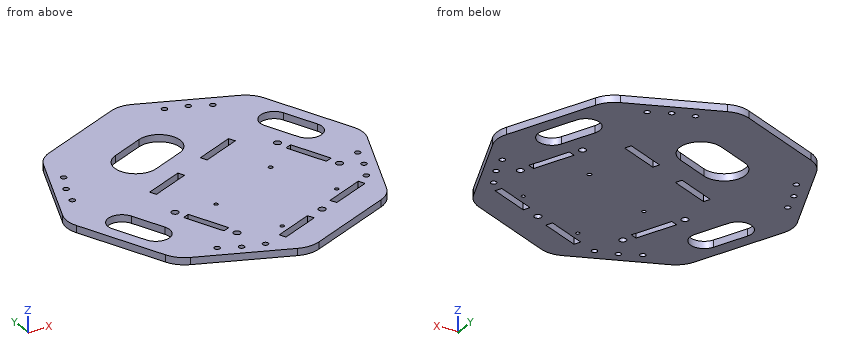
from build123d import *

# Parameters (mm, degrees)
SKETCH_1_R      = 2
SKETCH_1_R_2    = 2.5
SKETCH_1_R_3    = 1.35
SKETCH_1_R_4    = 1.5
EXTRUDE_1_DEPTH = 5
FILLET_1_R      = 20


with BuildPart() as part:
    # 草图1 → 凸台-拉伸1 (new body)
    with BuildSketch(Plane.XY):
        Polygon((0, 108.239220029), (-76.536686473, 76.536686473), (-108.239220029, 0), (-76.536686473, -76.536686473), (0, -108.239220029), (76.536686473, -76.536686473), (108.239220029, 0), (76.536686473, 76.536686473), align=None)
        with Locations((-35.206875778, -84.996916991)):
            Circle(SKETCH_1_R, mode=Mode.SUBTRACT)
        with Locations((84.996916991, -35.206875778)):
            Circle(SKETCH_1_R, mode=Mode.SUBTRACT)
        with Locations((35.206875778, 84.996916991)):
            Circle(SKETCH_1_R, mode=Mode.SUBTRACT)
        with Locations((-84.996916991, 35.206875778)):
            Circle(SKETCH_1_R, mode=Mode.SUBTRACT)
        with Locations((-45.41571145, -25.847352929)):
            Circle(SKETCH_1_R_2, mode=Mode.SUBTRACT)
        with Locations((-27.812273562, -68.345811425)):
            Circle(SKETCH_1_R_2, mode=Mode.SUBTRACT)
        with Locations((55.287157593, 15.865141198)):
            Circle(SKETCH_1_R_2, mode=Mode.SUBTRACT)
        with Locations((72.890595482, -26.633317297)):
            Circle(SKETCH_1_R_2, mode=Mode.SUBTRACT)
        with Locations((32.106246769, -70.586552674)):
            Circle(SKETCH_1_R_2, mode=Mode.SUBTRACT)
        with Locations((-18.756154363, -30.499289721)):
            Circle(SKETCH_1_R_3, mode=Mode.SUBTRACT)
        with Locations((-0.004666177, -75.769386814)):
            Circle(SKETCH_1_R_3, mode=Mode.SUBTRACT)
        with Locations((34.828858522, -8.303650644)):
            Circle(SKETCH_1_R_4, mode=Mode.SUBTRACT)
        with Locations((53.580346708, -53.573747737)):
            Circle(SKETCH_1_R_3, mode=Mode.SUBTRACT)
        with Locations((89.588318422, -20.926853617)):
            Circle(SKETCH_1_R, mode=Mode.SUBTRACT)
        with Locations((-20.926853617, -89.588318422)):
            Circle(SKETCH_1_R, mode=Mode.SUBTRACT)
        with Locations((-89.588318422, 20.926853617)):
            Circle(SKETCH_1_R, mode=Mode.SUBTRACT)
        with Locations((20.926853617, 89.588318422)):
            Circle(SKETCH_1_R, mode=Mode.SUBTRACT)
        with Locations((-48.55098737, -78.146027573)):
            Circle(SKETCH_1_R, mode=Mode.SUBTRACT)
        with Locations((-78.146027573, 48.55098737)):
            Circle(SKETCH_1_R, mode=Mode.SUBTRACT)
        with Locations((48.55098737, 78.146027573)):
            Circle(SKETCH_1_R, mode=Mode.SUBTRACT)
        with Locations((78.146027573, -48.55098737)):
            Circle(SKETCH_1_R, mode=Mode.SUBTRACT)
        Polygon((-40.04454516, -32.281680609), (-28.564042189, -59.998066584), (-33.183439852, -61.911483746), (-44.663942823, -34.19509777), align=None, mode=Mode.SUBTRACT)
        Polygon((-7.653402177, -84.349558002), (20.062983798, -72.869055031), (21.97640096, -77.488452694), (-5.739985015, -88.968955664), align=None, mode=Mode.SUBTRACT)
        Polygon((56.038926221, 7.517396357), (67.519429192, -20.198989618), (72.138826855, -18.285572456), (60.658323884, 9.430813519), align=None, mode=Mode.SUBTRACT)
        Polygon((-42.477594522, -0.276520543), (-14.761208547, 11.203982428), (-16.674625709, 15.82338009), (-44.391011684, 4.342877119), align=None, mode=Mode.SUBTRACT)
        Polygon((42.236092579, -63.684652654), (69.952478554, -52.204149683), (71.865895716, -56.823547346), (44.14950974, -68.304050317), align=None, mode=Mode.SUBTRACT)
        Polygon((7.411900233, 20.388384804), (35.128286209, 31.868887775), (33.214869047, 36.488285438), (5.498483072, 25.007782467), align=None, mode=Mode.SUBTRACT)
        with BuildLine():
            Line((-36.42291726, 55.268626709), (-13.325928947, 64.835712518))
            ThreePointArc((-13.325928947, 64.835712518), (6.272515526, 56.717771016), (-1.845425976, 37.119326542))
            Line((-1.845425976, 37.119326542), (-24.942414289, 27.552240733))
            ThreePointArc((-24.942414289, 27.552240733), (-44.540858762, 35.670182236), (-36.42291726, 55.268626709))
        make_face(mode=Mode.SUBTRACT)
        with BuildLine():
            Line((-70.32577989, -15.599989311), (-60.75869408, -38.696977624))
            ThreePointArc((-60.75869408, -38.696977624), (-66.170655082, -51.762607273), (-79.236284731, -46.350646271))
            Line((-79.236284731, -46.350646271), (-88.80337054, -23.253657958))
            ThreePointArc((-88.80337054, -23.253657958), (-83.391409538, -10.18802831), (-70.32577989, -15.599989311))
        make_face(mode=Mode.SUBTRACT)
        with BuildLine():
            Line((60.75869408, 38.696977624), (70.32577989, 15.599989311))
            ThreePointArc((70.32577989, 15.599989311), (83.391409538, 10.18802831), (88.80337054, 23.253657958))
            Line((88.80337054, 23.253657958), (79.236284731, 46.350646271))
            ThreePointArc((79.236284731, 46.350646271), (66.170655082, 51.762607273), (60.75869408, 38.696977624))
        make_face(mode=Mode.SUBTRACT)
    extrude(amount=EXTRUDE_1_DEPTH)

    # 圆角1
    fillet_1_edges = [part.edges().sort_by_distance(p)[0] for p in [
        (76.536686473, 76.536686473, 2.5),
        (108.239220029, 0, 2.5),
        (76.536686473, -76.536686473, 2.5),
        (0, -108.239220029, 2.5),
        (-76.536686473, -76.536686473, 2.5),
        (-108.239220029, 0, 2.5),
        (-76.536686473, 76.536686473, 2.5),
        (0, 108.239220029, 2.5),
    ]]
    fillet(fillet_1_edges, radius=FILLET_1_R)


solid = part.part
Source: CAD feature listing. Evaluate the final solid. Frame: model axes, mm. Round coordinates to 2 decimals unless told otherwise and drop trailing zeros. Loops run counter-clockwise (first coordinate to the right, second up) from the corner with the lowest first, then second, coordinate; pieces in that order, holes last. Notation, with made-up numbers: M 37,61.5 L 92,61.5 A18 ccw 92,68.5 Z; hole C 44.5,81.25 d4. An arc over 180 degrees is marked long. Answer as CSV lines item,"result".
Q1. Line query: line 1 along X through (y, z) = (-51, 4.5); line 2 along X through (y, z) = (-57.5, 2.9); line 3 along Y through (x, z) = (-21.5, 1.6). Output: solid intervals per line, ascending.
Verdict:
line 1,"x = -87.11 to -75.3, -64.69 to -37.7, -32.29 to 87.11"
line 2,"x = -84.42 to -35.01, -29.6 to 57.17, 70.23 to 84.42"
line 3,"y = -99.33 to -91.5, -87.67 to 8.41, 13.82 to 28.98, 61.45 to 99.33"
Q2. Cut plane B-B (z = 1.9). Count the separate pieces of the cut face and the enclosed holes in it, plus the area to 3 significant figures.
Verdict:
separate pieces,"1"
enclosed holes,"30"
area,"28,800 mm^2"
Q3. Cut plane A-A (x = 64). Return the cut outline in (y, z).
Verdict:
outline,"M -81.73,0 L -60.08,0 L -60.08,5 L -81.73,5 Z; M -54.67,0 L -11.7,0 L -11.7,5 L -54.67,5 Z; M 1.36,0 L 30.87,0 L 30.87,5 L 1.36,5 Z; M 50.53,0 L 81.73,0 L 81.73,5 L 50.53,5 Z"
Q4. Contact query for flat-ended pins moving along their axis: pin 1 (1.5 mm diameter, centred on y = 67.5, z = 3, fed in from -X); pin 2 (3 mm diameter, centred on x = 35.21, y = 85, fed in from +Z); pin 3 (1.5 mm diameter, centred on x = 66.5, z = 0.5, fed in from -Y); pin 4 (3 mm diameter, centred on y = -52.5, z = 1, fed in from +X). Output: stop coordinate, or through.
Verdict:
pin 1,"stops at x = -80.59"
pin 2,"passes through"
pin 3,"stops at y = -81"
pin 4,"stops at x = 87.11"
